from build123d import *

# Parameters (mm, degrees)
F1_DEPTH = 203.2
F3_DEPTH = 6.351


with BuildPart() as f1:
    # F0 (on Right) → F1 (new body)
    with BuildSketch(Plane.YZ):
        with BuildLine():
            Line((0, 95.25), (-6.35, 95.25))
            Line((-6.35, 95.25), (-6.35, 6.35))
            ThreePointArc((-6.35, 6.35), (-2.630256, -2.630256), (6.35, -6.35))
            Line((6.35, -6.35), (44.45, -6.35))
            Line((44.45, -6.35), (44.45, 0))
            Line((44.45, 0), (6.35, 0))
            ThreePointArc((6.35, 0), (1.859872, 1.859872), (0, 6.35))
            Line((0, 6.35), (0, 95.25))
        make_face()
    extrude(amount=F1_DEPTH)

    # F2 (on face) → F3 (cut, through all)
    with BuildSketch(Plane(origin=(0, 0, 0), x_dir=(-1, 0, 0), z_dir=(0, 1, 0))):
        with BuildLine():
            Line((-160.3375, 12.7), (-160.3375, 76.2))
            ThreePointArc((-160.3375, 76.2), (-165.1, 80.9625), (-169.8625, 76.2))
            Line((-169.8625, 76.2), (-169.8625, 12.7))
            ThreePointArc((-169.8625, 12.7), (-165.1, 7.9375), (-160.3375, 12.7))
        make_face()
        with BuildLine():
            Line((-33.3375, 12.7), (-33.3375, 76.2))
            ThreePointArc((-33.3375, 76.2), (-38.1, 80.9625), (-42.8625, 76.2))
            Line((-42.8625, 76.2), (-42.8625, 12.7))
            ThreePointArc((-42.8625, 12.7), (-38.1, 7.9375), (-33.3375, 12.7))
        make_face()
    extrude(amount=-F3_DEPTH, mode=Mode.SUBTRACT)


solid = f1.part
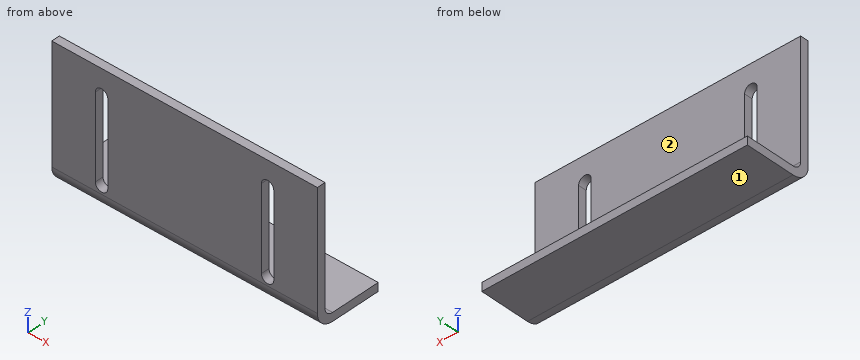
Input: part model. Units: mm. Frame: model coordinates. Face numbers are marked on the shaded views. A direction names the side the tool comes from. Coordinates: 2 decimals unless noted, no trailing zeros. Order: outer loops, then holes, each group sorted by start corner. A loop starts at its lowest first (then second) coordinate and runs counter-clockwise, first axis right, second up. Notation, with made-up numbers: M 40,2.5 L 95,2.5 A33 ccw 95,30.5 Z; hole C -34,69.25 d1. An arc over 180 degrees is marked long. Answer in a Markdown table with one row per item.
(1) Section query B-B, the plane x = 38.1. Output: boundary loops of the cut face in (y, z).
Numbers:
| item | result |
|---|---|
| outline | M -6.35,6.35 A12.7 ccw 6.35,-6.35 L 44.45,-6.35 L 44.45,0 L 6.35,0 A6.35 cw 0,6.35 L 0,7.94 L -6.35,7.94 Z; M -6.35,80.96 L 0,80.96 L 0,95.25 L -6.35,95.25 Z |
(2) Material intervals for line 1 (Y direction, x = 188, z = 18.5), sorted ascending. Write a range as [from, to].
Numbers:
| item | result |
|---|---|
| line 1 | y = [-6.35, 0] |
(3) Section query D-D, the plane y = -2.5. Give the number of separate pieces and of enclosed holes in the cut face, plus the area to 3 significant figures.
Numbers:
| item | result |
|---|---|
| separate pieces | 1 |
| enclosed holes | 2 |
| area | 18,600 mm^2 |
(4) Contact query for flat-ended pins moving along their axis: pin 1 Ø3 at (y, z) = (-4, 55.5) entering from -X; pin 2 Ø11.5 at (x, y) = (68.5, 33) entering from +Z. Output: stop coordinate, or through.
Numbers:
| item | result |
|---|---|
| pin 1 | stops at x = 0 |
| pin 2 | stops at z = 0 |
(5) Access query for the marked faces 1 and 2. Directions: +Z, -Z, +X, -X, +Y, -Y. A direction counts if a zero-diameter tool reaches every point of the face in a straight line with its end or side. Return the directions, or none.
Numbers:
| item | result |
|---|---|
| face 1 | -Z, +X, -X, +Y, -Y |
| face 2 | +Z, +X, -X, +Y |
(6) Section query C-C, the plane x = 97.5. Output: boundary loops of the cut face in (y, z).
Numbers:
| item | result |
|---|---|
| outline | M -6.35,6.35 A12.7 ccw 6.35,-6.35 L 44.45,-6.35 L 44.45,0 L 6.35,0 A6.35 cw 0,6.35 L 0,95.25 L -6.35,95.25 Z |
(7) Section query A-A, the plane z = 49.5. Output: boundary loops of the cut face in (x, y).
Numbers:
| item | result |
|---|---|
| outline | M 0,-6.35 L 33.34,-6.35 L 33.34,0 L 0,0 Z; M 42.86,-6.35 L 160.34,-6.35 L 160.34,0 L 42.86,0 Z; M 169.86,-6.35 L 203.2,-6.35 L 203.2,0 L 169.86,0 Z |
